Can you work these out from the model? Positions are in its coordinate system, mm. A direction names the side the tool comes from. Give positions to 0.01 mm unless a question says otherwise; leave off trailing zeros. Write each loop counter-clockwise with the first axis right and the second up, starting at its lowest first coordinate (ties: lowest second). Pieces come first, ordered by that corner, then holes.
from build123d import *

# Parameters (mm, degrees)
BOSS_EXTRUDE1_DEPTH = 10
RIB18_REACH         = 36.641
SKETCH15_WALL_W     = 95.323662864
SKETCH15_WALL_H     = 4.5
RIB38_REACH         = 36.641
SKETCH17_WALL_W     = 95.323662864
SKETCH17_WALL_H     = 4.5
BOSS_EXTRUDE2_DEPTH = 2.9
SKETCH36_R          = 5.25
CUT_EXTRUDE4_DEPTH  = 1
SKETCH37_R          = 3
CUT_EXTRUDE5_DEPTH  = 8
SKETCH33_R          = 5.25
CUT_EXTRUDE1_DEPTH  = 1
SKETCH38_R          = 3
CUT_EXTRUDE6_DEPTH  = 8


with BuildPart() as part:
    # Sketch2 → Boss-Extrude1 (new, symmetric)
    with BuildSketch(Plane(origin=(0, 0, 0), x_dir=(0, 0, -1), z_dir=(1, 0, 0))):
        Polygon((-20, 5), (-12, 5), (-12, -12), (5, -12), (5, -20), (-20, -20), align=None)
    extrude(amount=BOSS_EXTRUDE1_DEPTH, both=True)

    # Sketch15 wall → Rib18 (add, up to next)
    with BuildSketch(Plane(origin=(10, -3.5, 3.5), x_dir=(0, -0.707106781187, -0.707106781187), z_dir=(0, 0.707106781187, -0.707106781187)), mode=Mode.PRIVATE) as rib18_sk1:
        with Locations((0, 2.25)):
            Rectangle(SKETCH15_WALL_W, SKETCH15_WALL_H)
    rib18_tool1 = extrude(rib18_sk1.sketch, amount=-RIB18_REACH, mode=Mode.PRIVATE) - part.part
    add(rib18_tool1.solids().sort_by_distance((10, -3.5, 3.5))[0])

    # Sketch17 wall → Rib38 (add, up to next)
    with BuildSketch(Plane(origin=(-10, -3.5, 3.5), x_dir=(0, -0.707106781187, -0.707106781187), z_dir=(0, -0.707106781187, 0.707106781187)), mode=Mode.PRIVATE) as rib38_sk1:
        with Locations((0, 2.25)):
            Rectangle(SKETCH17_WALL_W, SKETCH17_WALL_H)
    rib38_tool1 = extrude(rib38_sk1.sketch, amount=RIB38_REACH, mode=Mode.PRIVATE) - part.part
    add(rib38_tool1.solids().sort_by_distance((-10, -3.5, 3.5))[0])

    # Sketch31 → Boss-Extrude2 (add, symmetric)
    with BuildSketch(Plane(origin=(0, 0, 0), x_dir=(0, 0, -1), z_dir=(1, 0, 0))):
        Polygon((-20, -10), (-20, -20), (-10, -20), (-13, -23), (-19.170777974, -23), (-23, -19.170777974), (-23, -13), align=None)
    extrude(amount=BOSS_EXTRUDE2_DEPTH, both=True)

    # Sketch36 → Cut-Extrude4 (cut)
    with BuildSketch(Plane(origin=(0, 0, 12), x_dir=(-1, 0, 0), z_dir=(0, 0, -1))):
        with Locations(Location((0, -1.5, 0), (0, 0, 90))):
            Circle(SKETCH36_R)
    extrude(amount=-CUT_EXTRUDE4_DEPTH, mode=Mode.SUBTRACT)

    # Sketch37 → Cut-Extrude5 (cut)
    with BuildSketch(Plane(origin=(0, 0, 13), x_dir=(-1, 0, 0), z_dir=(0, 0, -1))):
        with Locations(Location((0, -1.5, 0), (0, 0, 90))):
            Circle(SKETCH37_R)
    extrude(amount=-CUT_EXTRUDE5_DEPTH, mode=Mode.SUBTRACT)

    # Sketch33 → Cut-Extrude1 (cut)
    with BuildSketch(Plane(origin=(0, -12, 0), x_dir=(1, 0, 0), z_dir=(0, 1, 0))):
        with Locations(Location((0, -1.5, 0), (0, 0, 270))):
            Circle(SKETCH33_R)
    extrude(amount=-CUT_EXTRUDE1_DEPTH, mode=Mode.SUBTRACT)

    # Sketch38 → Cut-Extrude6 (cut)
    with BuildSketch(Plane(origin=(0, -13, 0), x_dir=(1, 0, 0), z_dir=(0, 1, 0))):
        with Locations(Location((0, -1.5, 0), (0, 0, 270))):
            Circle(SKETCH38_R)
    extrude(amount=-CUT_EXTRUDE6_DEPTH, mode=Mode.SUBTRACT)


solid = part.part
(1) For faces 3 (the face through (0, -7, 12)), 4 (the face through (3.55, -5.37, 12.49)), 5 (the face through (1.6, -12.5, 6.5)), which set-ups out of +Z, -Z, +X, -X, +Y, -Y let a thin tool reach every point of the face, with its end or its side?
Returned:
face 3: -Z, +Y
face 4: -Z
face 5: +Y
(2) Imagine slicing it at A-A, the plane z = 1.5. Write out the boundary of the cut face in (x, y).
Returned:
outline: (-10, -20) - (-3, -20) - (-3, -13) - (-5.25, -13) - (-5.25, -12) - (-5.5, -12) - (-5.5, -5.5) - (-10, -5.5) - close; (3, -20) - (10, -20) - (10, -5.5) - (5.5, -5.5) - (5.5, -12) - (5.25, -12) - (5.25, -13) - (3, -13) - close
(3) If I drill on L1, parallel to X at y = -15.75, z = 1.5; L2, parallel to X at y = -1.5, z = 12.75; L3, parallel to Z at x = 4.75, y = -2.5, over which ranges is the centre line in solid material (lowest first)?
Returned:
L1: x = -10 to -3, 3 to 10
L2: x = -10 to -5.25, 5.25 to 10
L3: z = 13 to 20
(4) If we mould it in two halves opening along X, with no side actions, what happens to faces 1 (the face through (0, -16, -5)), 2 (the face through (-2, 1, 13))? For each: +X half, -X half, draft (parallel to the pull), parting line (faces both ways), or undercut.
Returned:
face 1: draft
face 2: undercut
(5) Imagine slicing it at D-D, the plane y = -13.5. Write out the boundary of the cut face in (x, z).
Returned:
outline: (-10, -5) - (10, -5) - (10, 20) - (2.9, 20) - (2.9, 23) - (-2.9, 23) - (-2.9, 20) - (-10, 20) - close; hole circle Ø6 at (0, 1.5)
(6) Imagine slicing it at B-B, the plane y = -1.5. Write out the boundary of the cut face in (x, z).
Returned:
outline: (-10, 5.5) - (-5.5, 5.5) - (-5.5, 12) - (-5.25, 12) - (-5.25, 13) - (-3, 13) - (-3, 20) - (-10, 20) - close; (3, 13) - (5.25, 13) - (5.25, 12) - (5.5, 12) - (5.5, 5.5) - (10, 5.5) - (10, 20) - (3, 20) - close
(7) Will these pins go through, and if not, where does the flat tip stop? P1, Ø8, axis at x = 0, y = -1.5, coming from the -Z side; P2, Ø10, axis at x = -8, y = -11, coming from the -Z side; P3, Ø3, axis at x = -6, z = 8.5, coming from the +Y side; P4, Ø9, axis at x = 0, y = -4.5, coming from the -Z side.
Returned:
P1: stops at z = 13
P2: stops at z = -5
P3: stops at y = 3
P4: stops at z = 12
(8) Imagine slicing it at C-C, the plane x = 0. Write out the boundary of the cut face in (y, z), plus the area to 3 significant figures.
Returned:
outline: (-23, 13) - (-20, 10) - (-20, 4.5) - (-13, 4.5) - (-13, 6.75) - (-12, 6.75) - (-12, 12) - (-6.75, 12) - (-6.75, 13) - (-4.5, 13) - (-4.5, 20) - (-10, 20) - (-13, 23) - (-19.17, 23) - (-23, 19.17) - close; (-20, -5) - (-12, -5) - (-12, -3.75) - (-13, -3.75) - (-13, -1.5) - (-20, -1.5) - close; (1.5, 13) - (3.75, 13) - (3.75, 12) - (5, 12) - (5, 20) - (1.5, 20) - close
area: 284 mm2
